Could you check a few things on this model? Use its own coordinates, in mm. Face numbers are marked on the shaded views. A direction names the side the tool comes from. Give positions to 0.01 mm unless a question says otherwise; leave off trailing zeros. Order: outer loops, then holes, each group sorted by start corner. A loop starts at its lowest first (then second) coordinate and runs counter-clockwise, first axis right, second up. Notation, with made-up numbers: (24.25, 55.25) -> (28.25, 55.25) arc R21 cw to (28.25, 71.25) -> close; hole circle Ø5 at (-3, 48.25). An arc over 180 degrees is marked (long way). Answer as CSV lines item,"result". Start each with the question number.
(1) On a 3-axis mill with a long thin cutter (end or side, diameter ignored), from which of +Z, -Z, +X, -X, +Y, -Y can I reach the whole of each face in a straight line? I mean the marked faces 1 and 2. Say none if no direction works.
(2) I want a section at A-A (z = 88.9). Please give me the cut outline in (x, y).
(3) Will this pin go through, and if not, where does the flat tip stop? pin 1 Ø4 at (y, z) = (6.35, 177.8) entering from -X.
(4) I want a section at C-C (z = 177.8). Please give me the cut outline in (x, y).
(5) I want a section at B-B (x = -4.5). Please give me the cut outline in (y, z).
(6) I need wall thicknesses on L1, parallel to X at y = -0.25, z = 48; L2, parallel to Y at x = -12.1, z = 12.7. Which ranges of each line are inside material? Lowest first, please.
(7) We'd pull the mould along X, two halves only. Please class the marked faces 3, 4 and 5: released by +X, released by -X, zero draft, split by the parting line, or undercut.
```python
from build123d import *

# Parameters (mm, degrees)
BOSS_EXTRUDE1_DEPTH = 203.2
SKETCH2_R           = 3.429
SKETCH2_R_2         = 2.54
CUT_EXTRUDE1_DEPTH  = 26.4


with BuildPart() as part:
    # Sketch1 → Boss-Extrude1 (new body)
    with BuildSketch(Plane.XY):
        with BuildLine():
            Line((-12.446, -12.7), (12.446, -12.7))
            ThreePointArc((12.446, -12.7), (12.625605122, -12.625605122), (12.7, -12.446))
            Line((12.7, -12.446), (12.7, 12.446))
            ThreePointArc((12.7, 12.446), (12.625605122, 12.625605122), (12.446, 12.7))
            Line((12.446, 12.7), (-12.446, 12.7))
            ThreePointArc((-12.446, 12.7), (-12.625605122, 12.625605122), (-12.7, 12.446))
            Line((-12.7, 12.446), (-12.7, -12.446))
            ThreePointArc((-12.7, -12.446), (-12.625605122, -12.625605122), (-12.446, -12.7))
        make_face()
        with BuildLine():
            Line((-9.5885, 11.1125), (9.5885, 11.1125))
            ThreePointArc((9.5885, 11.1125), (10.666130735, 10.666130735), (11.1125, 9.5885))
            Line((11.1125, 9.5885), (11.1125, -9.5885))
            ThreePointArc((11.1125, -9.5885), (10.666130735, -10.666130735), (9.5885, -11.1125))
            Line((9.5885, -11.1125), (-9.5885, -11.1125))
            ThreePointArc((-9.5885, -11.1125), (-10.666130735, -10.666130735), (-11.1125, -9.5885))
            Line((-11.1125, -9.5885), (-11.1125, 9.5885))
            ThreePointArc((-11.1125, 9.5885), (-10.666130735, 10.666130735), (-9.5885, 11.1125))
        make_face(mode=Mode.SUBTRACT)
    extrude(amount=BOSS_EXTRUDE1_DEPTH)

    # Sketch2 → Cut-Extrude1 (cut, through all)
    with BuildSketch(Plane.ZY.offset(12.7)):
        with Locations((12.7, 0)):
            Circle(SKETCH2_R)
        with Locations((38.1, 0)):
            Circle(SKETCH2_R)
        with Locations((63.5, 0)):
            Circle(SKETCH2_R)
        with Locations((88.9, 0)):
            Circle(SKETCH2_R)
        with Locations((114.3, 0)):
            Circle(SKETCH2_R)
        with Locations((177.8, 6.35)):
            Circle(SKETCH2_R_2)
        with Locations((152.4, 6.35)):
            Circle(SKETCH2_R_2)
        with BuildLine():
            Line((6.35, 12.7), (0, 12.7))
            Line((0, 12.7), (0, 6.35))
            ThreePointArc((0, 6.35), (1.859871939, 10.840128061), (6.35, 12.7))
        make_face()
    extrude(amount=-CUT_EXTRUDE1_DEPTH, mode=Mode.SUBTRACT)


solid = part.part
```
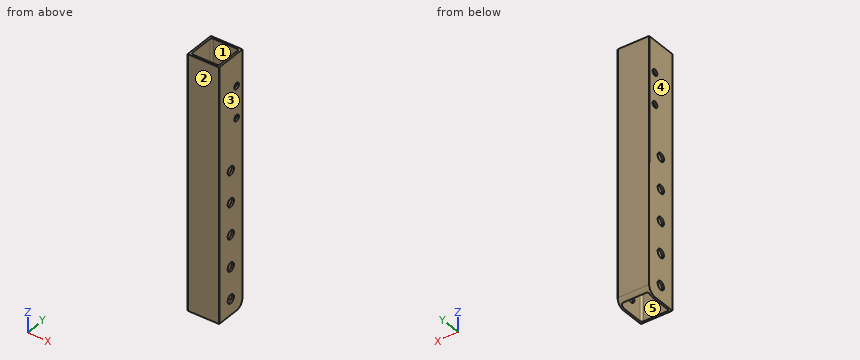
Final values:
1,face 1,"+Z, -Z"
1,face 2,"+Z, -Z, +X, -X, -Y"
2,outline,"(-12.7, -12.45) arc R0.25 ccw to (-12.45, -12.7) -> (12.45, -12.7) arc R0.25 ccw to (12.7, -12.45) -> (12.7, -3.43) -> (11.11, -3.43) -> (11.11, -9.59) arc R1.52 cw to (9.59, -11.11) -> (-9.59, -11.11) arc R1.52 cw to (-11.11, -9.59) -> (-11.11, -3.43) -> (-12.7, -3.43) -> close; (-12.7, 3.43) -> (-11.11, 3.43) -> (-11.11, 9.59) arc R1.52 cw to (-9.59, 11.11) -> (9.59, 11.11) arc R1.52 cw to (11.11, 9.59) -> (11.11, 3.43) -> (12.7, 3.43) -> (12.7, 12.45) arc R0.25 ccw to (12.45, 12.7) -> (-12.45, 12.7) arc R0.25 ccw to (-12.7, 12.45) -> close"
3,pin 1,"through"
4,outline,"(-12.7, -12.45) arc R0.25 ccw to (-12.45, -12.7) -> (12.45, -12.7) arc R0.25 ccw to (12.7, -12.45) -> (12.7, 3.81) -> (11.11, 3.81) -> (11.11, -9.59) arc R1.52 cw to (9.59, -11.11) -> (-9.59, -11.11) arc R1.52 cw to (-11.11, -9.59) -> (-11.11, 3.81) -> (-12.7, 3.81) -> close; (-12.7, 8.89) -> (-11.11, 8.89) -> (-11.11, 9.59) arc R1.52 cw to (-9.59, 11.11) -> (9.59, 11.11) arc R1.52 cw to (11.11, 9.59) -> (11.11, 8.89) -> (12.7, 8.89) -> (12.7, 12.45) arc R0.25 ccw to (12.45, 12.7) -> (-12.45, 12.7) arc R0.25 ccw to (-12.7, 12.45) -> close"
5,outline,"(-12.7, 0) -> (-11.11, 0) -> (-11.11, 203.2) -> (-12.7, 203.2) -> close; (11.11, 2.15) arc R6.35 ccw to (12.7, 6.35) -> (12.7, 203.2) -> (11.11, 203.2) -> close"
6,L1,"-12.7 to -11.11, 11.11 to 12.7"
6,L2,"-12.7 to -3.43, 3.43 to 12.7"
7,face 3,"released by +X"
7,face 4,"released by -X"
7,face 5,"undercut"
